Design review of the part built by this model. Coordinates are the model's own, in mm. A direction names the side the tool comes from. Round coordinates to 2 decimals unless told otherwise and drop trailing zeros. Loops run counter-clockwise (first coordinate to the right, second up) from the corner with the lowest first, then second, coordinate; pieces in that order, holes last. Notation, with made-up numbers: M 81.25,44.5 L 86.25,44.5 A11 cw 86.25,50.5 Z; hole C -7.75,-11 d5. An arc over 180 degrees is marked long. One line per item, written item: value. Start each with the question number.
Item 1: We need section C-C (y = 2.35). State how many separate pieces and enclosed holes the cut face has, then the cut area to 3 significant figures.
Item 2: For line 1 along X through (y, z) = (1.9, -7.62) (3 decimals); line 2 along Z through (x, y) = (1, 2.5); line 3 along X through (y, z) = (2.7, -37.86), list the stretches that pass through material, from the lowest coordinate up.
Item 3: We need section B-B (z = -30.86). Write out the cut boundary in (x, y) (3 decimals).
Item 4: Mouldability with a two-part tool opening along Z and no side actions: class faces 1 (the flat face through (15, 2, -14)), 2 (the cylindrical face through (13, 2, -42)), 3 (the flat face through (0, 2, 15)), 4 (the cylindrical face through (-8, 2, 5)) as released by +Z, released by -Z, zero draft, split by the parting line, or undercut.
Item 5: We need section A-A (x = -3.25). Write out the cut boundary in (y, z), then the cut area to 3 significant figures.
Item 6: Clearance check with a flat-ended pin moving along its axis: pin 1 (3 mm diameter, centred on x = 10, z = -37.86, fed in from +Y). State where the tip first meets the part, or that it passes through.
Item 7: For faces 5 (the flat face through (0, 2, -16.887)), 6 (the cylindrical face through (13, 2, 14)), list the 3-axis set-ups (+Z, -Z, +X, -X, +Y, -Y) from which the entire face can be reached by the end or side of a thin tool; tool diameter is ignored.
Item 8: We need section D-D (z = -19). Write out the cut boundary in (x, y), then the cut area to 3 significant figures.
from build123d import *

# Parameters (mm, degrees)
SKETCH1_W           = 30
SKETCH1_H           = 30
BOSS_EXTRUDE1_DEPTH = 4
SKETCH3_W           = 30
SKETCH3_H           = 28
BOSS_EXTRUDE2_DEPTH = 4
SKETCH2_R           = 0.95
SKETCH2_R_2         = 1.75
CUT_EXTRUDE1_DEPTH  = 46.716517803
FILLET1_R           = 5


with BuildPart() as part:
    # Sketch1 → Boss-Extrude1 (new body)
    with BuildSketch(Plane(origin=(0, 0, 0), x_dir=(1, 0, 0), z_dir=(0, 1, 0))):
        Rectangle(SKETCH1_W, SKETCH1_H)
    extrude(amount=BOSS_EXTRUDE1_DEPTH)

    # Sketch3 → Boss-Extrude2 (add)
    with BuildSketch(Plane(origin=(0, 4, 0), x_dir=(1, 0, 0), z_dir=(0, 1, 0))):
        with Locations((0, 29)):
            Rectangle(SKETCH3_W, SKETCH3_H)
    extrude(amount=-BOSS_EXTRUDE2_DEPTH)

    # Sketch2 → Cut-Extrude1 (cut, through all)
    with BuildSketch(Plane(origin=(0, 4, 0), x_dir=(1, 0, 0), z_dir=(0, 1, 0))):
        with Locations(Location((-10.795, -7.62, 0), (0, 0, 270))):
            Circle(SKETCH2_R)
        with Locations(Location((10.795, -7.62, 0), (0, 0, 270))):
            Circle(SKETCH2_R)
        with Locations(Location((10.795, 7.62, 0), (0, 0, 270))):
            Circle(SKETCH2_R)
        with Locations(Location((-10.795, 7.62, 0), (0, 0, 270))):
            Circle(SKETCH2_R)
        with Locations(Location((-10.795, 30.86, 0), (0, 0, 270))):
            Circle(SKETCH2_R)
        with Locations(Location((10.795, 30.86, 0), (0, 0, 270))):
            Circle(SKETCH2_R)
        with Locations(Location((10.795, 15.62, 0), (0, 0, 270))):
            Circle(SKETCH2_R)
        with Locations(Location((-10.795, 15.62, 0), (0, 0, 270))):
            Circle(SKETCH2_R)
        with Locations(Location((-10, 37.86, 0), (0, 0, 270))):
            Circle(SKETCH2_R_2)
        with Locations(Location((10, 37.86, 0), (0, 0, 270))):
            Circle(SKETCH2_R_2)
        with BuildLine():
            Line((-5, -6.352941176), (5, -6.352941176))
            ThreePointArc((5, -6.352941176), (7.828427125, -5.181368301), (9, -2.352941176))
            Line((9, -2.352941176), (9, 2.352941176))
            ThreePointArc((9, 2.352941176), (7.828427125, 5.181368301), (5, 6.352941176))
            Line((5, 6.352941176), (-5, 6.352941176))
            ThreePointArc((-5, 6.352941176), (-7.828427125, 5.181368301), (-9, 2.352941176))
            Line((-9, 2.352941176), (-9, -2.352941176))
            ThreePointArc((-9, -2.352941176), (-7.828427125, -5.181368301), (-5, -6.352941176))
        make_face()
        with BuildLine():
            Line((-5, 16.887058824), (5, 16.887058824))
            ThreePointArc((5, 16.887058824), (7.828427125, 18.058631699), (9, 20.887058824))
            Line((9, 20.887058824), (9, 25.592941176))
            ThreePointArc((9, 25.592941176), (7.828427125, 28.421368301), (5, 29.592941176))
            Line((5, 29.592941176), (-5, 29.592941176))
            ThreePointArc((-5, 29.592941176), (-7.828427125, 28.421368301), (-9, 25.592941176))
            Line((-9, 25.592941176), (-9, 20.887058824))
            ThreePointArc((-9, 20.887058824), (-7.828427125, 18.058631699), (-5, 16.887058824))
        make_face()
    extrude(amount=-CUT_EXTRUDE1_DEPTH, mode=Mode.SUBTRACT)

    # Fillet1
    fillet1_edges = [part.edges().sort_by_distance(p)[0] for p in [
        (15, 2, -43),
        (-15, 2, -43),
        (15, 2, 15),
        (-15, 2, 15),
    ]]
    fillet(fillet1_edges, radius=FILLET1_R)


solid = part.part
A:
1. separate pieces: 1
1. enclosed holes: 12
1. area: 1,250 mm2
2. line 1: -15 to -11.745, -9.845 to 9.845, 11.745 to 15
2. line 2: -43 to -29.59, -16.89 to -6.35, 6.35 to 15
2. line 3: -15 to -11.75, -8.25 to 8.25, 11.75 to 15
3. outline: M -15,0 L -11.745,0 L -11.745,4 L -15,4 Z; M -9.845,0 L 9.845,0 L 9.845,4 L -9.845,4 Z; M 11.745,0 L 15,0 L 15,4 L 11.745,4 Z
4. face 1: zero draft
4. face 2: released by -Z
4. face 3: released by +Z
4. face 4: undercut
5. outline: M 0,-43 L 4,-43 L 4,-29.59 L 0,-29.59 Z; M 0,-16.89 L 4,-16.89 L 4,-6.35 L 0,-6.35 Z; M 0,6.35 L 4,6.35 L 4,15 L 0,15 Z
5. area: 130 mm2
6. pin 1: through
7. face 5: +Y, -Y
7. face 6: +Z, +X, +Y, -Y
8. outline: M -15,0 L -8.53,0 L -8.53,4 L -15,4 Z; M 8.53,0 L 15,0 L 15,4 L 8.53,4 Z
8. area: 51.8 mm2
